The model under review builds one solid part; all positions refer to its coordinate system, in mm. Face numbers are marked on the shaded views. A direction names the side the tool comes from. Coordinates: 2 decimals unless noted, no trailing zeros. Loops run counter-clockwise (first coordinate to the right, second up) from the corner with the lowest first, then second, coordinate; pieces in that order, holes last. Notation, with made-up numbers: (-29, 57.5) - (25, 57.5) arc R24 ccw to (25, 96.5) - close; hole circle Ø3 at (52.5, -10). An arc over 180 degrees is marked (long way). One line per item, written item: value. Start each with the question number.
1. For the marked faces 1, 2 and 3, list the 3-axis set-ups (+Z, -Z, +X, -X, +Y, -Y) from which the entire face can be reached by the end or side of a thin tool; tool diameter is ignored.
2. To check wall thickness, follow line 1 (X direction, y = -5.5, z = 29); line 2 (Z direction, x = -1, y = -1.25). State the ranges of each line that lie inside material, in increasing order.
3. We need section B-B, the plane y = -1.5. Give the boundary of the cut face in (x, z).
4. Insertion check: P1, Ø11, axis at x = -2.5, z = 104.5, coming from the +Y side; P2, Ø5, axis at x = -3, z = 103, coming from the -Y side; P3, Ø3, axis at y = 2.5, z = 107, coming from the +X side. Each pin has a flat end and moves straight along its axis. Give the tip position at first contact, or say it passes through.
5. We need section D-D, the plane z = 103.5. Give the boundary of the cut face in (x, y), then the cut area to 3 significant figures.
6. Mouldability with a two-part tool opening along X and no side actions: class the marked faces 4, 5, 6 and 7 as +X half, -X half, draft (parallel to the pull), parting line (faces both ways), or undercut.
7. We need section A-A, the plane z = 49. Give the boundary of the cut face in (x, y).
from build123d import *

# Parameters (mm, degrees)
SKETCH_1_W          = 20
SKETCH_1_H          = 20
EXTRUDE_1_DEPTH     = 100
SKETCH_3_W          = 18
SKETCH_3_H          = 18
EXTRUDE_2_DEPTH     = 10
SKETCH_4_W          = 16
SKETCH_4_H          = 16
CUT_EXTRUDE_1_DEPTH = 100


with BuildPart() as part:
    # 草圖1 → 填料-伸長1 (new body)
    with BuildSketch(Plane.XY):
        Rectangle(SKETCH_1_W, SKETCH_1_H)
    extrude(amount=EXTRUDE_1_DEPTH)

    # 草圖3 → 填料-伸長2 (add)
    with BuildSketch(Plane.XY.offset(100)):
        Rectangle(SKETCH_3_W, SKETCH_3_H)
    extrude(amount=EXTRUDE_2_DEPTH)

    # 草圖4 → 除料-伸長1 (cut)
    with BuildSketch(Plane.XY.offset(110)):
        Rectangle(SKETCH_4_W, SKETCH_4_H)
    extrude(amount=-CUT_EXTRUDE_1_DEPTH, mode=Mode.SUBTRACT)


solid = part.part
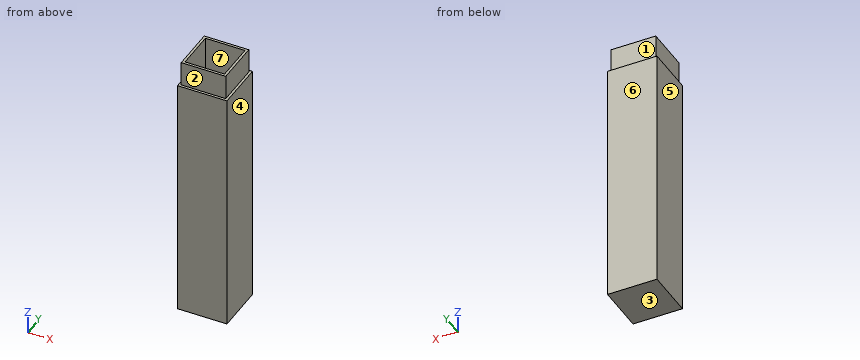
Findings below:
1. face 1: +Z, +X, -X, +Y
1. face 2: +Z, +X, -X, -Y
1. face 3: -Z, +X, -X, +Y, -Y
2. line 1: -10 to -8, 8 to 10
2. line 2: 0 to 10
3. outline: (-10, 0) - (10, 0) - (10, 100) - (9, 100) - (9, 110) - (8, 110) - (8, 10) - (-8, 10) - (-8, 110) - (-9, 110) - (-9, 100) - (-10, 100) - close
4. P1: y = 10
4. P2: y = -9
4. P3: x = 9
5. outline: (-9, -9) - (9, -9) - (9, 9) - (-9, 9) - close; hole (-8, -8) - (8, -8) - (8, 8) - (-8, 8) - close
5. area: 68.0 mm2
6. face 4: +X half
6. face 5: -X half
6. face 6: draft
6. face 7: undercut
7. outline: (-10, -10) - (10, -10) - (10, 10) - (-10, 10) - close; hole (-8, -8) - (8, -8) - (8, 8) - (-8, 8) - close
